Can you work these out from the model? Positions are in its coordinate system, mm. A direction names the side the tool comes from. Round coordinates to 2 decimals unless told otherwise and drop trailing zeros. Loops run counter-clockwise (first coordinate to the right, second up) from the corner with the lowest first, then second, coordinate; pieces in that order, holes last. Notation, with made-up numbers: M 67.5,83 L 99.5,83 A23 cw 99.5,96 Z; hole C 47.5,-34.5 d9. An arc over 180 degrees is marked long. Return JSON: item names as keys, results as strings.
```python
from build123d import *

# Parameters (mm, degrees)
SKETCH001_R     = 76.835
POCKET_DEPTH    = 3.175
SKETCH002_W     = 114
SKETCH002_H     = 90
POCKET001_DEPTH = 5
SKETCH003_W     = 14
SKETCH003_H     = 14
POCKET002_DEPTH = 16.826
SKETCH004_W     = 28.4
SKETCH004_H     = 28.4
POCKET003_DEPTH = 9
SKETCH005_W     = 35.5
SKETCH005_H     = 7
POCKET004_DEPTH = 3
FILLET_R        = 12.7
SKETCH006_R     = 2
POCKET005_DEPTH = 5


with BuildPart() as part:
    # Sketch → Revolution (revolve)
    with BuildSketch(Plane.XZ):
        Polygon((0, 5), (0, 20), (80, 20), (80, 5), (77.5, -5), (75.5, -5), (75.5, 0), (75.5, 5), align=None)
    revolve(axis=Axis((0, 0, 0), (0, 0, 1)))

    # Sketch001 (on Face1 of Revolution) → Pocket (cut)
    with BuildSketch(Plane(origin=(0, 0, 20), x_dir=(-1, 0, 0), z_dir=(0, 0, 1))):
        Circle(SKETCH001_R)
    extrude(amount=-POCKET_DEPTH, mode=Mode.SUBTRACT)

    # Sketch002 (on Face5 of Pocket) → Pocket001 (cut)
    with BuildSketch(Plane(origin=(0, 0, 16.825), x_dir=(-1, 0, 0), z_dir=(0, 0, 1))):
        Rectangle(SKETCH002_W, SKETCH002_H)
    extrude(amount=-POCKET001_DEPTH, mode=Mode.SUBTRACT)

    # Sketch003 (on Face12 of Pocket001) → Pocket002 (cut, through all)
    with BuildSketch(Plane(origin=(0, 0, 11.825), x_dir=(-1, 0, 0), z_dir=(0, 0, 1))):
        with Locations((0, 35)):
            Rectangle(SKETCH003_W, SKETCH003_H)
    extrude(amount=-POCKET002_DEPTH, mode=Mode.SUBTRACT)

    # Sketch004 (on Face5 of Pocket002) → Pocket003 (cut)
    with BuildSketch(Plane(origin=(0, 0, 16.825), x_dir=(-1, 0, 0), z_dir=(0, 0, 1))):
        with Locations((0, -59.2)):
            Rectangle(SKETCH004_W, SKETCH004_H)
    extrude(amount=-POCKET003_DEPTH, mode=Mode.SUBTRACT)

    # Sketch005 (on Face5 of Pocket003) → Pocket004 (cut)
    with BuildSketch(Plane(origin=(0, 0, 16.825), x_dir=(-1, 0, 0), z_dir=(0, 0, 1))):
        with Locations((-31.95, -48.5)):
            Rectangle(SKETCH005_W, SKETCH005_H)
    extrude(amount=-POCKET004_DEPTH, mode=Mode.SUBTRACT)

    # Fillet
    fillet_edges = [part.edges().sort_by_distance(p)[0] for p in [
        (57, -45, 14.325),
        (57, 45, 14.325),
        (-57, -45, 14.325),
        (-57, 45, 14.325),
    ]]
    fillet(fillet_edges, radius=FILLET_R)

    # Sketch006 (on Face17 of Fillet) → Pocket005 (cut)
    with BuildSketch(Plane(origin=(0, 0, 11.825), x_dir=(-1, 0, 0), z_dir=(0, 0, 1))):
        with Locations((-49.6, 38)):
            Circle(SKETCH006_R)
        with Locations((49.6, 38)):
            Circle(SKETCH006_R)
        with Locations((-49.6, -36.2)):
            Circle(SKETCH006_R)
        with Locations((49.6, -36.2)):
            Circle(SKETCH006_R)
    extrude(amount=-POCKET005_DEPTH, mode=Mode.SUBTRACT)


solid = part.part
```
Q1. On a 3-axis mill with a long thin cutter (end or side, diameter ignored), from which of +Z, -Z, +X, -X, +Y, -Y can I reach the whole of each face in a straight line? I mean faces 1 (the flat face through (7, -35, 8)), 2 (the flat face through (-14.2, 59, 12)). Say none if no direction works.
Results:
{"face 1": "+Z, -Z", "face 2": "+Z"}
Q2. Suppose I cut it at B-B, the plane y = 0. Please give me the cut outline in (x, z) (3 decimals), plus the area to 3 significant figures.
Results:
{"outline": "M -80,5 L -77.5,-5 L -75.5,-5 L -75.5,5 L 75.5,5 L 75.5,-5 L 77.5,-5 L 80,5 L 80,20 L 76.835,20 L 76.835,16.825 L 57,16.825 L 57,11.825 L -57,11.825 L -57,16.825 L -76.835,16.825 L -76.835,20 L -80,20 Z", "area": "1,410 mm2"}
Q3. I'm going to push flat-ended pins straight in: pin 1 Ø3 at (x, y) = (49.6, -38) entering from -Z; pin 2 Ø0.9 at (x, z) = (31, 15.5) entering from -Y; pin 3 Ø10 at (x, y) = (7, -56) entering from +Z (3 decimals). Where does each tip first touch, or does it pass through?
Results:
{"pin 1": "stops at z = 5", "pin 2": "stops at y = -73.94", "pin 3": "stops at z = 16.825"}
Q4. If I drill on line 1 along Y through (x, z) = (49.6, 8.5); line 2 along X through (y, z) = (36.2, 8.85); line 3 along X through (y, z) = (-9, 15.75), over which ranges is the centre line in solid material (lowest first)?
Results:
{"line 1": "y = -62.77 to -40, -36 to 34.2, 38.2 to 62.77", "line 2": "x = -71.34 to -51.6, -47.6 to 47.6, 51.6 to 71.34", "line 3": "x = -79.49 to -57, 57 to 79.49"}
Q5. Suppose I cut it at A-A, the plane x = 0. Please give me the cut outline in (y, z) (3 decimals).
Results:
{"outline": "M -80,5 L -77.5,-5 L -75.5,-5 L -75.5,5 L -42,5 L -42,11.825 L -45,11.825 L -45,16.825 L -76.835,16.825 L -76.835,20 L -80,20 Z; M -28,5 L 75.5,5 L 75.5,-5 L 77.5,-5 L 80,5 L 80,20 L 76.835,20 L 76.835,16.825 L 73.4,16.825 L 73.4,7.825 L 45,7.825 L 45,11.825 L -28,11.825 Z"}
